Can you work these out from the model? Positions are in its coordinate system, mm. A direction names the side the tool comes from. Round coordinates to 2 decimals unless told otherwise and drop trailing zeros. Loops run counter-clockwise (first coordinate to the right, second up) from the corner with the lowest first, then second, coordinate; pieces in that order, holes last. Notation, with made-up numbers: (24.5, 34.25) -> (75.5, 34.25) arc R16 ccw to (75.5, 58.25) -> close; hole circle Ø2 at (-7, 28.25). An arc over 180 degrees is marked (long way). Write each question's results on one line, items separated by ' | '.
from build123d import *

# Parameters (mm, degrees)
F1_DEPTH = 254
F2_SIZE  = 19.04999
F3_W     = 63.5
F3_H     = 19.05
F4_DEPTH = 6.35
F5_R     = 3.175


# Not quite as in the source:
# - a fillet or chamfer is up to 0.001 mm smaller than in the source, because OpenCascade refuses the exact size


with BuildPart() as f1:
    # F0 (on Front) → F1 (new body)
    with BuildSketch(Plane.XZ):
        Polygon((203.2, 9.525), (-203.2, 9.525), (-184.15, -9.525), (184.15, -9.525), align=None)
    extrude(amount=-F1_DEPTH)

    # F2 (size 19.05 in the source; OpenCascade refuses exactly that, so slightly less here)
    f2_edges = [f1.edges().sort_by_distance(p)[0] for p in [
        (0, 254, -9.525),
    ]]
    chamfer(f2_edges, length=F2_SIZE)

    # F3 (on face) → F4 (cut)
    with BuildSketch(Plane(origin=(0, 0, -9.525), x_dir=(1, 0, 0), z_dir=(0, 0, -1))):
        with Locations((-152.4, -28.575)):
            Rectangle(F3_W, F3_H)
        with Locations((31.75, -28.575)):
            Rectangle(F3_W, F3_H)
        with Locations((31.75, -206.375)):
            Rectangle(F3_W, F3_H)
        with Locations((-152.4, -206.375)):
            Rectangle(F3_W, F3_H)
    extrude(amount=-F4_DEPTH, mode=Mode.SUBTRACT)

    # F5
    f5_edges = [f1.edges().sort_by_distance(p)[0] for p in [
        (0, 0, 9.525),
        (0, 0, -9.525),
    ]]
    fillet(f5_edges, radius=F5_R)


solid = f1.part
1. If we section it at B-B (y = 208): List the corners of the cut face in (x, z) for me (3 decimals).
Final values:
outline: (-203.2, 9.525) -> (-184.15, -9.525) -> (-184.15, -3.175) -> (-120.65, -3.175) -> (-120.65, -9.525) -> (0, -9.525) -> (0, -3.175) -> (63.5, -3.175) -> (63.5, -9.525) -> (184.15, -9.525) -> (203.2, 9.525) -> close
2. Will these pins go through, and if not, where does the flat tip stop? pin 1 (5.5 mm diameter, centred on x = -158, y = 24, fed in from -Z) (3 decimals); pin 2 (3 mm diameter, centred on y = 205.5, z = -7.5, fed in from +X) (3 decimals); pin 3 (1.5 mm diameter, centred on y = 145.5, z = 6, fed in from +X) (3 decimals); pin 4 (7 mm diameter, centred on x = -164, z = -7.5, fed in from -Y).
Final values:
pin 1: z = -3.175 | pin 2: x = 187.675 | pin 3: x = 200.425 | pin 4: y = 0
3. On a 3-axis mill with a long thin cutter (end or side, diameter ignored), from which of +Z, -Z, +X, -X, +Y, -Y can I reach the whole of each face in a straight line? I mean faces 1 (the face through (-153, 28, -3.175)), 2 (the face through (-2.845, 244.608, 0.133)). Say none if no direction works.
Final values:
face 1: -Z | face 2: -Z, +X, -X, +Y
4. Please list where these lines run through material, in increasing order: line 1 (Y direction, x = -127, z = -3.25) (3 decimals); line 2 (Z direction, x = -127, y = 32) (3 decimals); line 3 (Y direction, x = -177.5, z = -8.5) (3 decimals). Write a range as from..to.
Final values:
line 1: 0..19.05, 38.1..196.85, 215.9..241.225 | line 2: -3.175..9.525 | line 3: 0.839..19.05, 38.1..196.85, 215.9..235.975
5. We'd pull the mould along Y, two halves only. Please class faces 3 (the face through (-3, 0, 0)), 4 (the face through (-153, 206, -3.175)), 5 (the face through (-193.808, 125.222, 0.133)): pulls with the +Y half, pulls with the -Y half, needs draft (parallel to the pull), parting line crosses it, or undercut.
Final values:
face 3: pulls with the -Y half | face 4: undercut | face 5: needs draft
6. If we section it at D-D (z = 0.5): List the corners of the cut face in (x, y) for me (3 decimals).
Final values:
outline: (-194.175, 0) -> (194.175, 0) -> (194.175, 244.975) -> (-194.175, 244.975) -> close
